Part model, mm, in its own coordinate system. A direction names the side the tool comes from. Give positions to 0.01 mm unless a question says otherwise; leave off trailing zeros. Order: outer loops, then holes, each group sorted by start corner. A loop starts at its lowest first (then second) coordinate and runs counter-clockwise, first axis right, second up. Notation, with made-up numbers: M 54.5,-3.5 L 61.5,-3.5 A23 cw 61.5,15.5 Z; hole C -8,35 d6. An arc over 180 degrees is marked long. Return JSON: item names as keys, results as strings.
from build123d import *

# Parameters (mm, degrees)
SKETCH1_R           = 3
BOSS_EXTRUDE1_DEPTH = 5
BOSS_EXTRUDE2_DEPTH = 8


with BuildPart() as part:
    # Sketch1 → Boss-Extrude1 (new body)
    with BuildSketch(Plane(origin=(0, 0, 0), x_dir=(1, 0, 0), z_dir=(0, 1, 0))):
        with Locations(Location((0, 0, 0), (0, 0, 270))):
            Circle(SKETCH1_R)
    extrude(amount=BOSS_EXTRUDE1_DEPTH)

    # Sketch2 → Boss-Extrude2 (add)
    with BuildSketch(Plane.XZ):
        Polygon((1.35, -2.33826859), (1.35, 2.33826859), (-2.7, 0), align=None)
    extrude(amount=BOSS_EXTRUDE2_DEPTH)


solid = part.part
Q1. 3-axis set-ups, long thin cutter, end or side, ignore diameter. For faces 1 (the flat face through (-0.703, -3.944, -1.153)), 2 (the flat face through (-0.647, -3.944, 1.186)), 3 (the flat face through (1.35, -4, 0)): which of +Z, -Z, +X, -X, +Y, -Y reach the whole face in a straight line?
Established:
{"face 1": "-Z, -X, -Y", "face 2": "+Z, -X, -Y", "face 3": "+Z, -Z, +X, -Y"}
Q2. Band-saw the part on D-D (y = 1.5). Give the cut face in (x, z).
Established:
{"outline": "C 0,0 d6"}
Q3. Probe line 1 along Y through (x, z) = (1.5, -2.25); line 2 along Z through (x, y) = (-0.55, -6.5); line 3 along Z through (x, y) = (0.9, -3.5). List the from-to ranges inside material, lowest first.
Established:
{"line 1": "y = 0 to 5", "line 2": "z = -1.24 to 1.24", "line 3": "z = -2.08 to 2.08"}
Q4. Band-saw the part on B-B (y = -3). Give the cut face in (x, z), then the cut area to 3 significant figures.
Established:
{"outline": "M -2.7,0 L 1.35,-2.34 L 1.35,2.34 Z", "area": "9.47 mm²"}
Q5. Pin check, flat tips, straight feed: pin 1 (1.5 mm diameter, centred on y = -5.5, z = -2, fed in from -X); pin 2 (3 mm diameter, centred on x = 1.5, y = -4, fed in from -Z); pin 3 (2 mm diameter, centred on y = 3.5, z = 2.5, fed in from -X). Stop position of each tip, or through.
Established:
{"pin 1": "stops at x = -0.53", "pin 2": "stops at z = -2.34", "pin 3": "stops at x = -2.6"}
Q6. Band-saw the part on C-C (z = -1.5). Give the cut face in (x, y).
Established:
{"outline": "M -2.6,0 L -0.1,0 L -0.1,-8 L 1.35,-8 L 1.35,0 L 2.6,0 L 2.6,5 L -2.6,5 Z"}
Q7. Band-saw the part on A-A (x = 0). Give the cut face in (y, z), then the cut area to 3 significant figures.
Established:
{"outline": "M -8,-1.56 L 0,-1.56 L 0,-3 L 5,-3 L 5,3 L 0,3 L 0,1.56 L -8,1.56 Z", "area": "54.9 mm²"}
